Can you work these out from the model? Positions are in its coordinate system, mm. Face numbers are marked on the shaded views. A direction names the side the tool comes from. Round coordinates to 2 decimals unless told otherwise and drop trailing zeros. Loops run counter-clockwise (first coordinate to the right, second up) from the corner with the lowest first, then second, coordinate; pieces in that order, holes last.
(1) I want a section at D-D on x = 133.5. Write out the boundary of the cut face in (y, z), plus the area to 3 significant figures.
(2) If I drill on line 1 along Z through (x, y) = (19.45, 1.85) (3 decimals); line 2 along X through (y, z) = (1.4, 90.84); line 3 along X through (y, z) = (0.8, 15), over which ranges is the centre line in solid material (lowest first)?
(3) Which directions (+Z, -Z, +X, -X, +Y, -Y) give clear straight access to the entire face, cutting with the end or side of a thin tool? Please do the marked faces 4 and 5.
(4) I want a section at A-A on z = 80. Write out the boundary of the cut face in (x, y), plus the area to 3 significant figures.
(5) Thinking about a two-plate mould opening in X: for the marked faces 1, 2 and 3, which applies, released by +X, released by -X, zero draft, split by the parting line, or undercut?
(6) Will these pins go through, and if not, where does the flat tip stop? pin 1 Ø2.5 at (x, z) = (164.5, 6) entering from +Y; pin 2 Ø1.5 at (x, z) = (72.5, 92) entering from +Y.
(7) I want a section at B-B on y = 11. Write out the boundary of the cut face in (x, z).
(8) I want a section at C-C on z = 47.5. Write out the boundary of the cut face in (x, y), plus the area to 3 significant figures.
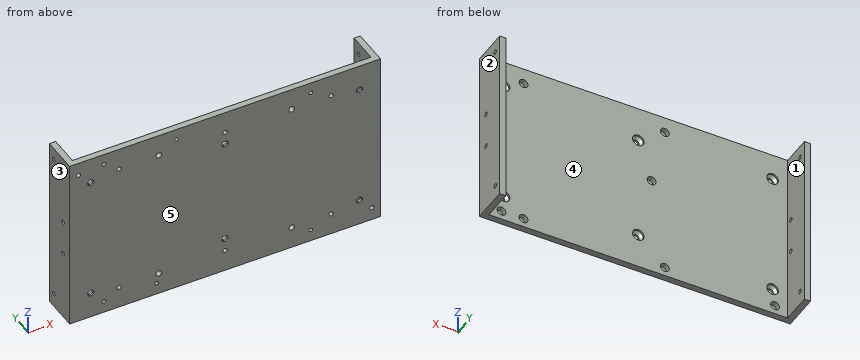
from build123d import *

# Parameters (mm, degrees)
EXTRUDE_1_DEPTH              = 100
HOLE_WIZARD_2_5_2_5_1_D      = 2.5
HOLE_WIZARD_2_5_2_5_1_DEPTH  = 3
HOLE_WIZARD_M2_51_D          = 2.05
HOLE_WIZARD_M2_51_DEPTH      = 3
HOLE_WIZARD_M31_D            = 2.5
HOLE_WIZARD_M31_DEPTH        = 3
HOLE_WIZARD_M41_D            = 3.3
HOLE_WIZARD_M41_DEPTH        = 3
HOLE_WIZARD_M32_D            = 2.5
HOLE_WIZARD_M32_DEPTH        = 3.5
HOLE_WIZARD_M33_D            = 2.5
HOLE_WIZARD_M33_DEPTH        = 5.5
HOLE_WIZARD_M31_2_AT_2_COUNT = 2
HOLE_WIZARD_M31_2_AT_2_PITCH = 76.164296097
HOLE_WIZARD_M31_2_AT_3_COUNT = 2
HOLE_WIZARD_M31_2_AT_3_PITCH = 152
HOLE_WIZARD_M31_2_AT_4_COUNT = 2
HOLE_WIZARD_M31_2_AT_4_PITCH = 70
HOLE_WIZARD_M31_2_AT_5_COUNT = 2
HOLE_WIZARD_M31_2_AT_5_PITCH = 100.004999875
HOLE_WIZARD_M31_2_AT_6_COUNT = 2
HOLE_WIZARD_M31_2_AT_6_PITCH = 167.343957166
HOLE_WIZARD_5_0_5_1_D        = 5
HOLE_WIZARD_5_0_5_1_DEPTH    = 3


with BuildPart() as part:
    # Эскиз1 → Вытянуть-Тонкостенный1 (new body)
    with BuildSketch(Plane.XY):
        Polygon((0, 20.7), (0, 0), (176, 0), (176, 20.7), (172.5, 20.7), (172.5, 3.5), (3.5, 3.5), (3.5, 20.7), align=None)
    extrude(amount=EXTRUDE_1_DEPTH)

    # Диаметр отверстия Ø2.5 (2.5)1
    with Locations(Plane(origin=(0, 0, 0), x_dir=(-1, 0, 0), z_dir=(0, -1, 0))):
        with Locations((-5, -92.5), (-171, -7.5)):
            Hole(HOLE_WIZARD_2_5_2_5_1_D / 2, depth=HOLE_WIZARD_2_5_2_5_1_DEPTH)

    # Отверстие обработанное метчиком M2,51
    with Locations(Plane(origin=(0, 0, 0), x_dir=(-1, 0, 0), z_dir=(0, -1, 0))):
        with Locations((-19.45, -93.75), (-60.45, -93.75), (-136.45, -93.75), (-136.45, -6.75), (-49.25, -6.75), (-19.45, -6.75)):
            Hole(HOLE_WIZARD_M2_51_D / 2, depth=HOLE_WIZARD_M2_51_DEPTH)

    # Hole Wizard M31
    with Locations(Plane(origin=(0, 0, 0), x_dir=(-1, 0, 0), z_dir=(0, -1, 0))):
        with Locations((-28, -87.5), (-88, -87.5), (-148, -87.5), (-148, -12.5), (-88, -12.5), (-28, -12.5)):
            Hole(HOLE_WIZARD_M31_D / 2, depth=HOLE_WIZARD_M31_DEPTH)

    # Отверстие обработанное метчиком M41
    with Locations(Plane(origin=(0, 0, 0), x_dir=(-1, 0, 0), z_dir=(0, -1, 0))):
        with Locations((-50.5, -87.5), (-125.7, -87.5), (-125.7, -12.5), (-50.5, -12.5)):
            Hole(HOLE_WIZARD_M41_D / 2, depth=HOLE_WIZARD_M41_DEPTH)

    # Отверстие обработанное метчиком M32
    with Locations(Plane(origin=(176, 0, 0), x_dir=(0, 0, -1), z_dir=(1, 0, 0))):
        with Locations((-93, 16.2), (-60, 6.7), (-40, 6.7), (-8, 16.2)):
            Hole(HOLE_WIZARD_M32_D / 2, depth=HOLE_WIZARD_M32_DEPTH)

    # Отверстие обработанное метчиком M33
    with Locations(Plane.ZY):
        with Locations((93, 16.2), (60, 6.7), (40, 6.7), (8, 16.2)):
            Hole(HOLE_WIZARD_M33_D / 2, depth=HOLE_WIZARD_M33_DEPTH)

    # Эскиз14 → Hole Wizard M31 2 (revolve, cut)
    with BuildSketch(Plane(origin=(12, 3.5, 15), x_dir=(0, 0, 1), z_dir=(1, 0, 0))):
        Polygon((0, 0), (0, 3.5), (1.8, 3.5), (1.8, 2.5), (3.3, 1), (3.3, 0), align=None)
    hole_wizard_m31_2 = revolve(axis=Axis((12, 9.85, 15), (0, -1, 0)), mode=Mode.SUBTRACT)

    # Hole Wizard M31 2 at 2: Hole Wizard M31 2 ×2
    with Locations(*[Vector(0.9978428725040861, 0, 0.06564755740158466) * (i * HOLE_WIZARD_M31_2_AT_2_PITCH) for i in range(1, HOLE_WIZARD_M31_2_AT_2_COUNT)]):
        add(hole_wizard_m31_2, mode=Mode.SUBTRACT)

    # Hole Wizard M31 2 at 3: Hole Wizard M31 2 ×2
    with Locations(*[(i * HOLE_WIZARD_M31_2_AT_3_PITCH, 0, 0) for i in range(1, HOLE_WIZARD_M31_2_AT_3_COUNT)]):
        add(hole_wizard_m31_2, mode=Mode.SUBTRACT)

    # Hole Wizard M31 2 at 4: Hole Wizard M31 2 ×2
    with Locations(*[(0, 0, i * HOLE_WIZARD_M31_2_AT_4_PITCH) for i in range(1, HOLE_WIZARD_M31_2_AT_4_COUNT)]):
        add(hole_wizard_m31_2, mode=Mode.SUBTRACT)

    # Hole Wizard M31 2 at 5: Hole Wizard M31 2 ×2
    with Locations(*[Vector(0.7599620028497626, 0, 0.649967502437297) * (i * HOLE_WIZARD_M31_2_AT_5_PITCH) for i in range(1, HOLE_WIZARD_M31_2_AT_5_COUNT)]):
        add(hole_wizard_m31_2, mode=Mode.SUBTRACT)

    # Hole Wizard M31 2 at 6: Hole Wizard M31 2 ×2
    with Locations(*[Vector(0.9083088662063591, 0, 0.41830013575292857) * (i * HOLE_WIZARD_M31_2_AT_6_PITCH) for i in range(1, HOLE_WIZARD_M31_2_AT_6_COUNT)]):
        add(hole_wizard_m31_2, mode=Mode.SUBTRACT)

    # Диаметр отверстия Ø5.0 (5)1
    with Locations(Plane(origin=(0, 3.5, 0), x_dir=(1, 0, 0), z_dir=(0, 1, 0))):
        with Locations((165.42, -5.05), (152.97, -5.12), (72.96, -5.12), (10.58, -5.05), (80.5, -57.25), (72.96, -90.84), (152.97, -90.84)):
            Hole(HOLE_WIZARD_5_0_5_1_D / 2, depth=HOLE_WIZARD_5_0_5_1_DEPTH)


solid = part.part
Filled sheet:
1. outline: (0, 0) - (3.5, 0) - (3.5, 100) - (0, 100) - close
1. area: 350 mm2
2. line 1: z = 0 to 5.725, 7.775 to 92.725, 94.775 to 100
2. line 2: x = 0 to 70.46, 75.46 to 150.47, 155.47 to 176
2. line 3: x = 0 to 10.2, 13.8 to 162.2, 165.8 to 176
3. face 4: +Z, -Z, +Y
3. face 5: +Z, -Z, +X, -X, -Y
4. outline: (0, 0) - (86.2, 0) - (86.2, 1) - (84.7, 2.5) - (84.7, 3.5) - (3.5, 3.5) - (3.5, 20.7) - (0, 20.7) - close; (89.8, 0) - (176, 0) - (176, 20.7) - (172.5, 20.7) - (172.5, 3.5) - (91.3, 3.5) - (91.3, 2.5) - (89.8, 1) - close
4. area: 719 mm2
5. face 1: undercut
5. face 2: released by +X
5. face 3: released by -X
6. pin 1: stops at y = 3.5
6. pin 2: stops at y = 0.5
7. outline: (0, 0) - (3.5, 0) - (3.5, 100) - (0, 100) - close; (172.5, 0) - (176, 0) - (176, 100) - (172.5, 100) - close
8. outline: (0, 0) - (176, 0) - (176, 20.7) - (172.5, 20.7) - (172.5, 3.5) - (3.5, 3.5) - (3.5, 20.7) - (0, 20.7) - close
8. area: 736 mm2
